from build123d import *

# Parameters (mm, degrees)
SKETCH1_R               = 21.55
SKETCH1_R_2             = 16.55
BOSS_EXTRUDE1_DEPTH     = 5
CUT_EXTRUDE2_DEPTH      = 15
CUT_EXTRUDE2_DEPTH_BACK = 12


with BuildPart() as part:
    # Sketch1 → Boss-Extrude1 (new body)
    with BuildSketch(Plane(origin=(0, 0, 0), x_dir=(1, 0, 0), z_dir=(0, 1, 0))):
        Circle(SKETCH1_R)
        Circle(SKETCH1_R_2, mode=Mode.SUBTRACT)
    extrude(amount=BOSS_EXTRUDE1_DEPTH)

    # Sketch3 → Cut-Extrude2 (cut, two sides)
    with BuildSketch(Plane(origin=(0, 0, 0), x_dir=(1, 0, 0), z_dir=(0, 1, 0))) as cut_extrude2_sk:
        Polygon((-1.758392575, -22.689237535), (2.305538937, -22.689237535), (0.504822735, -15.993131255), (0, -15.993131255), (-0.488859737, -15.993131255), align=None)
    extrude(amount=CUT_EXTRUDE2_DEPTH, mode=Mode.SUBTRACT)
    extrude(cut_extrude2_sk.sketch, amount=-CUT_EXTRUDE2_DEPTH_BACK, mode=Mode.SUBTRACT)


solid = part.part
Build history of the part. All positions in model axes, mm. Coordinates: 2 decimals unless noted, no trailing zeros. Order: outer loops, then holes, each group sorted by start corner. A loop starts at its lowest first (then second) coordinate and runs counter-clockwise, first axis right, second up. Notation, with made-up numbers: (-15, 28.5) - (42, 28.5) arc R27 cw to (42, 63.5) - close; hole circle Ø5 at (20.5, 29). An arc over 180 degrees is marked (long way). Write each question's results on one line, items separated by ' | '. Start each with the question number.
Item 1: Band-saw the part on B-B on z = 15. Write the cut outline in (x, y).
Item 2: Band-saw the part on C-C on x = 0. Write the cut outline in (y, z), and give its area (3 significant figures).
Item 3: Flat gauge pin, fed straight in: pin 1 (12 mm diameter, centred on x = -15.5, z = 12, fed in from -Y). Where does the tip first touch, or does it go through?
Item 4: Band-saw the part on A-A on z = -3. Write the cut outline in (x, y).
Item 5: Band-saw the part on D-D on y = 2.15. Write the cut outline in (x, z).
Item 6: Mould opens along X. For faces 1 (the face through (0.7, 2.46, -21.54)), 2 (the face through (16, 5, -5)), 3 (the face through (-1.056, 2.465, 18.983)), 4 (the face through (1.32, 2.46, 19.03)) say: released by +X, released by -X, zero draft, split by the parting line, or undercut.
Item 7: Wall check: probe 1 along X at (y, z) = (3.35, 0); probe 2 along Z at (x, y) = (0, 1.15); probe 3 along Z at (x, y) = (-14, 2.05). Give the ranges that are in metal, low to high. Write a range as [from, to].
Numbers:
1) outline: (-15.47, 0) - (-6.99, 0) - (-6.99, 5) - (-15.47, 5) - close; (6.99, 0) - (15.47, 0) - (15.47, 5) - (6.99, 5) - close
2) outline: (0, -21.55) - (5, -21.55) - (5, -16.55) - (0, -16.55) - close | area: 25.0 mm^2
3) pin 1: y = 0
4) outline: (-21.34, 0) - (-16.28, 0) - (-16.28, 5) - (-21.34, 5) - close; (16.28, 0) - (21.34, 0) - (21.34, 5) - (16.28, 5) - close
5) outline: (-1.53, 21.5) arc R21.55 ccw (long way) to (1.97, 21.46) - (0.65, 16.54) arc R16.55 cw (long way) to (-0.59, 16.54) - close
6) face 1: split by the parting line | face 2: zero draft | face 3: undercut | face 4: undercut
7) probe 1: [-21.55, -16.55], [16.55, 21.55] | probe 2: [-21.55, -16.55] | probe 3: [-16.38, -8.83], [8.83, 16.38]
